from build123d import *

# Parameters (mm, degrees)
CUT_EXTRUDE1_START           = -4
CUT_EXTRUDE1_DEPTH           = 4
F_3_0_3_DIAMETER_HOLE1_D     = 3
M2_CLEARANCE_HOLE1_REACH     = 69.343
M2_CLEARANCE_HOLE1_BORE_R    = 1.2645
F_2_0_2_DIAMETER_HOLE1_D     = 2
F_2_0_2_DIAMETER_HOLE1_DEPTH = 1.631966011
M2_CLEARANCE_HOLE2_D         = 2.529
M2_CLEARANCE_HOLE2_DEPTH     = 5.5
M2_CLEARANCE_HOLE3_D         = 2.529
M2_CLEARANCE_HOLE3_DEPTH     = 6.035533906
CHAMFER1_SIZE                = 0.2
FILLET1_R                    = 1


with BuildPart() as part:
    # Sketch1 → Revolve1 (revolve)
    with BuildSketch(Plane.XZ, mode=Mode.PRIVATE) as revolve1_sk:
        Polygon((1.7, 11.75), (0, 11.75), (0, -55.5), (2.5, -55.5), (2.5, 0), (2, 0), (2, 0.75), (2.5, 0.75), (2.5, 10.364359354), align=None)
    revolve(revolve1_sk.sketch.rotate(Axis((0, 0, 11.75), (0, 0, -1)), 180), axis=Axis((0, 0, 11.75), (0, 0, -1)))

    # Sketch2 → Cut-Extrude1 (cut)
    with BuildSketch(Plane(origin=(0, 0, -52.5), x_dir=(-1, 0, 0), z_dir=(0, 0, -1)).offset(CUT_EXTRUDE1_START)):
        with BuildLine():
            Line((1.5, -2), (-1.5, -2))
            ThreePointArc((-1.5, -2), (0, -2.5), (1.5, -2))
        make_face()
    extrude(amount=CUT_EXTRUDE1_DEPTH, mode=Mode.SUBTRACT)

    # Ø3.0 (3) Diameter Hole1 (through all)
    with Locations(Plane(origin=(0, -2.5, 7.75), x_dir=(-1, 0, 0), z_dir=(0, -1, 0))):
        with Locations((0, 0)):
            Hole(F_3_0_3_DIAMETER_HOLE1_D / 2)

    # M2 Clearance Hole1 bore → M2 Clearance Hole1 (cut, up to next)
    with BuildSketch(Plane.XY.offset(11.75), mode=Mode.PRIVATE) as m2_clearance_hole1_sk1:
        Circle(M2_CLEARANCE_HOLE1_BORE_R)
    m2_clearance_hole1_tool1 = extrude(m2_clearance_hole1_sk1.sketch, amount=-M2_CLEARANCE_HOLE1_REACH, mode=Mode.PRIVATE) & part.part
    add(m2_clearance_hole1_tool1.solids().sort_by_distance((0, 0, 11.75))[0], mode=Mode.SUBTRACT)

    # Ø2.0 (2) Diameter Hole1
    with Locations(Plane.XY.offset(6.631966011)):
        with Locations((0, 0)):
            Hole(F_2_0_2_DIAMETER_HOLE1_D / 2, depth=F_2_0_2_DIAMETER_HOLE1_DEPTH)

    # M2 Clearance Hole2
    with Locations(Plane(origin=(0, 0, -55.5), x_dir=(-1, 0, 0), z_dir=(0, 0, -1))):
        with Locations((0, 0)):
            Hole(M2_CLEARANCE_HOLE2_D / 2, depth=M2_CLEARANCE_HOLE2_DEPTH)

    # M2 Clearance Hole3
    with Locations(Plane(origin=(1.767766953, -1.767766953, -26), x_dir=(0.707106781187, 0.707106781187, 0), z_dir=(0.707106781187, -0.707106781187, 0))):
        with Locations((0, 0)):
            Hole(M2_CLEARANCE_HOLE3_D / 2, depth=M2_CLEARANCE_HOLE3_DEPTH)

    # Chamfer1
    chamfer1_edges = [part.edges().sort_by_distance(p)[0] for p in [
        (2.5, 0, -55.5),
    ]]
    chamfer(chamfer1_edges, length=CHAMFER1_SIZE)

    # Fillet1
    fillet1_edges = [part.edges().sort_by_distance(p)[0] for p in [
        (2.5, 0, 10.364359354),
    ]]
    fillet(fillet1_edges, radius=FILLET1_R)


solid = part.part
The listing builds one solid part. Answer for the finished solid, in the listing's coordinates (mm). A direction names the side the tool comes from. Round coordinates to 2 decimals unless told otherwise and drop trailing zeros. Write each loop counter-clockwise with the first axis right and the second up, starting at its lowest first coordinate (ties: lowest second). Pieces come first, ordered by that corner, then holes. Notation, with made-up numbers: (33, 58) - (42, 58) arc R7 ccw to (42, 71) - close; hole circle Ø6 at (27, 41.5). An arc over 180 degrees is marked (long way). Use one line per item in the form item = value. Start each with the question number.
Item 1: Find the intervals of material crossed by line 1 (Z direction, x = 0.35, y = -0.6); line 2 (Y direction, x = 0, z = -52.25); line 3 (Z direction, x = 0, y = 1.55), in increasing order. Write a range as [from, to].
Item 2: A cutting plane is placed at C-C (z = -18.5). Write down the section's boundary in (x, y), plus the area to 3 significant figures.
Item 3: A cutting plane is placed at A-A (z = 7.75). Write down the section's boundary in (x, y), plus the area to 3 significant figures.
Item 4: Determine the mould class of faces 1 (the cylindrical face through (0.434, -1.952, 0.38)), 2 (the flat face through (0, 0, 5)), 3 (the flat face through (0, -2, -55.5)) for opening direction Z: +Z half, -Z half, draft (parallel to the pull), parting line (faces both ways), or undercut.
Item 5: Flat-ended cylindrical pins translate along their axes: pin 1 Ø1.5 at (x, z) = (0, -50.5) entering from -Y; pin 2 Ø1.5 at (y, z) = (2, -45) entering from +X; pin 3 Ø1 at (x, z) = (-1.5, -8) entering from +Y. Find the tip coordinate at first contact, or state that the pin passes through.
Item 6: A cutting plane is placed at B-B (x = 0). Give the number of separate pieces and of enclosed holes in the cut face, plus the area to 3 significant figures.
Item 7: A tool of negligible diameter and unlimited length cuts with its end or side. For faces 4 (the flat face through (0, 0, -50)), 5 (the flat face through (0, -2, -50)), 6 (the cylindrical face through (-1.11, 0.04, 6.74)), 7 (the flat face through (1, 2, 0)), 8 (the cylindrical face through (0.68, 1.066, 10.176)), from which of +Z, -Z, +X, -X, +Y, -Y can it reach the whole face along a straight path? Write none if from no direction.
The answers:
q1.line_1 = [-50, -27.25], [-24.75, 5]
q1.line_2 = [-2, -1.26], [1.26, 2.5]
q1.line_3 = [-55.5, -26.63], [-25.37, 6.25], [9.25, 11.75]
q2.outline = circle Ø5 at (0, 0)
q2.area = 19.6 mm^2
q3.outline = (-1.5, -2) - (-1.5, 2) arc R2.5 ccw to start; (1.5, -2) arc R2.5 ccw to (1.5, 2) - close
q3.area = 5.59 mm^2
q4.face_1 = undercut
q4.face_2 = +Z half
q4.face_3 = -Z half
q5.pin_1 = -2
q5.pin_2 = 2.17
q5.pin_3 = 2.29
q6.separate_pieces = 3
q6.enclosed_holes = 1
q6.area = 288 mm^2
q7.face_4 = -Z
q7.face_5 = +X, -X, -Y
q7.face_6 = +Y, -Y
q7.face_7 = none
q7.face_8 = +Z
